Source: CAD feature listing. Evaluate the final solid. Frame: model axes, mm. Face numbers are marked on the shaded views. A direction names the side the tool comes from. Round coordinates to 2 decimals unless told otherwise and drop trailing zeros. Order: outer loops, then holes, each group sorted by start corner. A loop starts at its lowest first (then second) coordinate and runs counter-clockwise, first axis right, second up. Notation, with made-up numbers: (-14.75, 60.25) - (12.25, 60.25) arc R17 ccw to (12.25, 65.25) - close; hole circle Ø10 at (-0.5, 6.25). An arc over 180 degrees is marked (long way). Put each result on its own line as item: value. Start each with the question number.
1) Line query: probe 1 along X at (y, z) = (2.75, 3.5); probe 2 along Y at (x, z) = (20, 1.1); probe 3 along Y at (x, z) = (20, 3.05). Output: solid intervals per line, ascending. Write a range as [from, to].
2) Section A-A on z = 8.25. Output: boundary loops of the cut face in (x, y), then the cut area to 3 significant figures.
3) Section C-C on y = 4.5. Output: boundary loops of the cut face in (x, z), then the cut area to 3 significant figures.
4) Section D-D on x = -52.5. Output: boundary loops of the cut face in (y, z), then the cut area to 3 significant figures.
5) Mould query, pull axis X, two halves, no side actions, for the marked faces 4, 5, 6 and 7. Classes: +X half, -X half, draft (parallel to the pull), parting line (faces both ways), or undercut.
6) Contact query for flat-ended pins moving along their axis: P1, Ø7.5, axis at x = -0.5, y = 2.5, coming from the +Z side; P2, Ø8, axis at x = -5.5, y = -6.5, coming from the -Z side; P3, Ø6, axis at x = 20, y = -0.5, coming from the +Z side; P4, Ø11.5, axis at x = 52, z = 16, coming from the -Y side. Output: stop coordinate, or through.
7) Section B-B on x = 48.5. Output: boundary loops of the cut face in (y, z), then the cut area to 4 significant figures.
8) Access query for the marked faces 1, 2 and 3. Directions: +Z, -Z, +X, -X, +Y, -Y. A direction counts if a zero-diameter tool reaches every point of the face in a straight line with its end or side. Return the directions, or none.
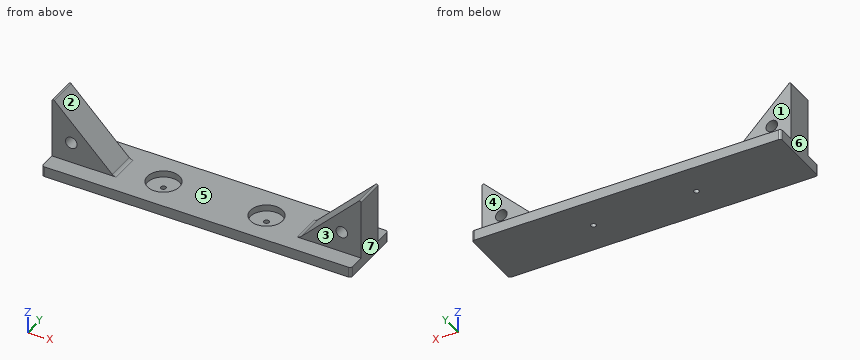
```python
from build123d import *

# Parameters (mm, degrees)
SKETCH_W        = 120
SKETCH_H        = 25
PAD_DEPTH       = 4
SKETCH001_R     = 2.25
PAD001_DEPTH    = 5.7
FILLET_R        = 2
FILLET001_R     = 0.5
FILLET002_R     = 1
SKETCH002_R     = 6.25
POCKET_DEPTH    = 2.5
SKETCH003_R     = 1
POCKET001_DEPTH = 1.501


with BuildPart() as part:
    # Sketch → Pad (new body)
    with BuildSketch(Plane.XY):
        Rectangle(SKETCH_W, SKETCH_H)
    extrude(amount=PAD_DEPTH)

    # Sketch001 → Pad001 (join, symmetric)
    with BuildSketch(Plane.XZ):
        Polygon((-60, 4), (-60, 28), (-36, 4), align=None)
        with Locations((-52.5, 12)):
            Circle(SKETCH001_R, mode=Mode.SUBTRACT)
        Polygon((60, 4), (36, 4), (60, 28), align=None)
        with Locations((52.5, 12)):
            Circle(SKETCH001_R, mode=Mode.SUBTRACT)
    extrude(amount=PAD001_DEPTH, both=True)

    # Fillet
    fillet_edges = [part.edges().sort_by_distance(p)[0] for p in [
        (-36, 0, 4),
        (36, 0, 4),
    ]]
    fillet(fillet_edges, radius=FILLET_R)

    # Fillet001
    fillet001_edges = [part.edges().sort_by_distance(p)[0] for p in [
        (-60, 0, 28),
        (60, 0, 28),
    ]]
    fillet(fillet001_edges, radius=FILLET001_R)

    # Fillet002
    fillet002_edges = [part.edges().sort_by_distance(p)[0] for p in [
        (-60, 12.5, 2),
        (-60, -12.5, 2),
        (60, -12.5, 2),
        (60, 12.5, 2),
    ]]
    fillet(fillet002_edges, radius=FILLET002_R)

    # Sketch002 (on Face1 of Fillet002) → Pocket (cut)
    with BuildSketch(Plane.XY.offset(4)):
        with Locations((-20, 0)):
            Circle(SKETCH002_R)
        with Locations((20, 0)):
            Circle(SKETCH002_R)
    extrude(amount=-POCKET_DEPTH, mode=Mode.SUBTRACT)

    # Sketch003 (on Face27 of Pocket) → Pocket001 (cut, through all)
    with BuildSketch(Plane.XY.offset(1.5)):
        with Locations((-20, 0)):
            Circle(SKETCH003_R)
        with Locations((20, 0)):
            Circle(SKETCH003_R)
    extrude(amount=-POCKET001_DEPTH, mode=Mode.SUBTRACT)


solid = part.part
```
Answer sheet:
1. probe 1: [-60, -25.61], [-14.39, 14.39], [25.61, 60]
1. probe 2: [-12.5, -1], [1, 12.5]
1. probe 3: [-12.5, -6.25], [6.25, 12.5]
2. outline: (-60, -5.7) - (-40.25, -5.7) - (-40.25, 5.7) - (-60, 5.7) - close; (40.25, -5.7) - (60, -5.7) - (60, 5.7) - (40.25, 5.7) - close
2. area: 450 mm^2
3. outline: (-60, 0) - (60, 0) - (60, 26.79) arc R0.5 ccw to (59.15, 27.15) - (36.59, 4.59) arc R2 cw to (35.17, 4) - (24.34, 4) - (24.34, 1.5) - (15.66, 1.5) - (15.66, 4) - (-15.66, 4) - (-15.66, 1.5) - (-24.34, 1.5) - (-24.34, 4) - (-35.17, 4) arc R2 cw to (-36.59, 4.59) - (-59.15, 27.15) arc R0.5 ccw to (-60, 26.79) - close; hole circle Ø4.5 at (-52.5, 12); hole circle Ø4.5 at (52.5, 12)
3. area: 980 mm^2
4. outline: (-12.5, 0) - (12.5, 0) - (12.5, 4) - (5.7, 4) - (5.7, 9.75) - (-5.7, 9.75) - (-5.7, 4) - (-12.5, 4) - close; (-5.7, 14.25) - (5.7, 14.25) - (5.7, 20.5) - (-5.7, 20.5) - close
4. area: 237 mm^2
5. face 4: draft
5. face 5: undercut
5. face 6: -X half
5. face 7: +X half
6. P1: z = 4
6. P2: z = 0
6. P3: z = 1.5
6. P4: y = -5.7
7. outline: (-12.5, 0) - (12.5, 0) - (12.5, 4) - (5.7, 4) - (5.7, 16.5) - (-5.7, 16.5) - (-5.7, 4) - (-12.5, 4) - close
7. area: 242.5 mm^2
8. face 1: +Z, +X, -X, +Y
8. face 2: +Z, +Y, -Y
8. face 3: +Z, +X, -X, -Y
